CAD build for the part. Positions are in the model's coordinates, mm. Face numbers are marked on the shaded views. Coordinates: 2 decimals unless noted, no trailing zeros. Loops run counter-clockwise (first coordinate to the right, second up) from the corner with the lowest first, then second, coordinate; pieces in that order, holes last. Notation, with made-up numbers: (51.25, -37) -> (109.25, -37) arc R18 ccw to (109.25, -29) -> close; hole circle Ø5 at (-38, -24). An arc over 180 degrees is marked (long way). Answer as a JSON object with one key per item and string values. Group by question number.
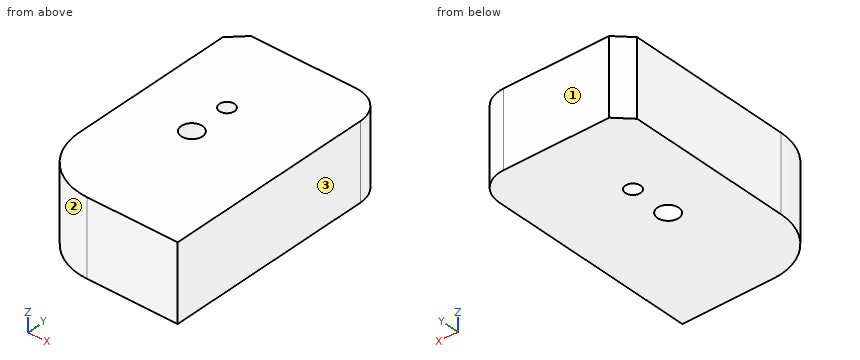
from build123d import *

# Parameters (mm, degrees)
F0_W     = 50
F0_H     = 80
F1_DEPTH = 25
F2_R     = 10
F3_SIZE  = 5
F4_R     = 20
F5_R     = 2.5
F5_R_2   = 3.5
F6_DEPTH = 30


with BuildPart() as f1:
    # F0 (on Top) → F1 (new body)
    with BuildSketch(Plane.XY):
        with Locations((25, -40)):
            Rectangle(F0_W, F0_H)
    extrude(amount=F1_DEPTH)

    # F2
    f2_edges = [f1.edges().sort_by_distance(p)[0] for p in [
        (50, 0, 12.5),
    ]]
    fillet(f2_edges, radius=F2_R)

    # F3
    f3_edges = [f1.edges().sort_by_distance(p)[0] for p in [
        (0, 0, 12.5),
    ]]
    chamfer(f3_edges, length=F3_SIZE)

    # F4
    f4_edges = [f1.edges().sort_by_distance(p)[0] for p in [
        (0, -80, 12.5),
    ]]
    fillet(f4_edges, radius=F4_R)

    # F5 (on face) → F6 (cut)
    with BuildSketch(Plane(origin=(0, 0, 0), x_dir=(1, 0, 0), z_dir=(0, 0, -1))):
        with Locations((20.888399, 27.508826)):
            Circle(F5_R)
        with Locations((20.965385, 41.043077)):
            Circle(F5_R_2)
    extrude(amount=-F6_DEPTH, mode=Mode.SUBTRACT)


solid = f1.part
Item 1: Drill centre lines: L1, parallel to Y at x = 23, z = 24; L2, parallel to Y at x = 20.5, z = 21; L3, parallel to X at y = -9.5, z = 16.5. Where is each one in solid material? Low to high.
Item 2: Band-saw the part on C-C, the plane y = -69.5. List the corners of the cut face in (x, z).
Item 3: Flat gauge pin, fed straight in: P1, Ø8, axis at x = 14, z = 14, coming from the -Y side. Where does the tip first touch, or does it go through?
Item 4: Band-saw the part on B-B, the plane x = 12. List the corners of the cut face in (y, z).
Item 5: Pull direction X, two halves, no side cores. Call the marked faces 1, 2 and 3: +X half, -X half, draft (parallel to the pull), parting line (faces both ways), or undercut.
Item 6: Band-saw the part on A-A, the plane z = 21.25. List the corners of the cut face in (x, y), and give its area (3 significant figures).
Reply:
{
 "1": {"L1": "-80 to -43.89, -38.2 to -28.85, -26.17 to 0", "L2": "-80 to -44.51, -37.57 to -29.98, -25.04 to 0", "L3": "0 to 49.99"},
 "2": {"outline": "(2.4, 0) -> (50, 0) -> (50, 25) -> (2.4, 25) -> close"},
 "3": {"P1": "y = -79.9"},
 "4": {"outline": "(-78.33, 0) -> (0, 0) -> (0, 25) -> (-78.33, 25) -> close"},
 "5": {"face 1": "draft", "face 2": "-X half", "face 3": "+X half"},
 "6": {"outline": "(0, -60) arc R20 ccw to (20, -80) -> (50, -80) -> (50, -10) arc R10 ccw to (40, 0) -> (5, 0) -> (0, -5) -> close; hole circle Ø7 at (20.97, -41.04); hole circle Ø5 at (20.89, -27.51)", "area": "3,820 mm²"}
}
